Input: part model. Units: mm. Frame: model coordinates. Face numbers are marked on the shaded views. A direction names the side the tool comes from. Coordinates: 2 decimals unless noted, no trailing zeros. Order: outer loops, then holes, each group sorted by start corner. A loop starts at its lowest first (then second) coordinate and runs counter-clockwise, first axis right, second up. Notation, with made-up numbers: (47.25, -37.75) - (78.25, -37.75) arc R13 ccw to (78.25, -12.75) - close; hole circle Ø8 at (44, 9). An arc over 180 degrees is marked (long way). Use a Markdown table: item, result. Add a question column.
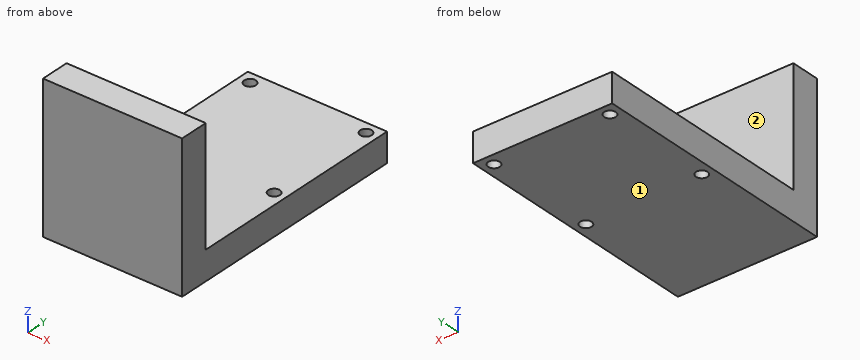
from build123d import *

# Parameters (mm, degrees)
SKETCH3_W           = 48
SKETCH3_H           = 30
SKETCH3_H_2         = 47
SKETCH3_R           = 2
SKETCH3_H_3         = 10
BOSS_EXTRUDE1_DEPTH = 10
SKETCH3_3_W         = 48
SKETCH3_3_H         = 10
BOSS_EXTRUDE2_DEPTH = 50


with BuildPart() as part:
    # Sketch3 → Boss-Extrude1 (new body)
    # profile 1 of 3: a face of its own
    with BuildSketch(Plane.XY):
        with Locations((0, -38.5)):
            Rectangle(SKETCH3_W, SKETCH3_H)
    # profile 2 of 3: a face of its own
    with BuildSketch(Plane.XY):
        Rectangle(SKETCH3_W, SKETCH3_H_2)
        with Locations((-20, 19.5)):
            Circle(SKETCH3_R, mode=Mode.SUBTRACT)
        with Locations((-20, -19.5)):
            Circle(SKETCH3_R, mode=Mode.SUBTRACT)
        with Locations((20, -19.5)):
            Circle(SKETCH3_R, mode=Mode.SUBTRACT)
        with Locations((20, 19.5)):
            Circle(SKETCH3_R, mode=Mode.SUBTRACT)
    # profile 3 of 3: a face of its own
    with BuildSketch(Plane.XY):
        with Locations((0, -58.5)):
            Rectangle(SKETCH3_W, SKETCH3_H_3)
    extrude(amount=BOSS_EXTRUDE1_DEPTH)

    # Sketch3_3 → Boss-Extrude2 (add)
    with BuildSketch(Plane.XY):
        with Locations((0, -58.5)):
            Rectangle(SKETCH3_3_W, SKETCH3_3_H)
    extrude(amount=BOSS_EXTRUDE2_DEPTH)


solid = part.part
1) Cut plane B-B (y = -19.5). Return the cut outline in (x, z).
2) Cut plane C-C (x = -7.5). Return the cut outline in (y, z), and give its area (3 significant figures).
3) Cut plane A-A (x = -20). Return the cut outline in (y, z), and give its area (3 significant figures).
4) Reachability of the marked faces 1 and 2 from +Z, -Z, +X, -X, +Y, -Y: full face, straight path, thin tool, end or side. Return the list, or none.
5) Material intervals for L1, parallel to Y at x = -20, z = 3.5; L2, parallel to X at y = 19, z = 4; L3, parallel to Z at x = -1.5, y = -50.5, sorted ascending.
6) Cut plane D-D (z = 38). Return the cut outline in (x, y), and give its area (3 significant figures).
7) Contact query for flat-ended pins moving along their axis: P1, Ø3, axis at x = 12.5, y = -54, coming from the -Z side; P2, Ø5, axis at x = 18, y = -13.5, coming from the +Z side; P3, Ø20, axis at x = 5.5, z = 37.5, coming from the +Y side; P4, Ø3.5, axis at x = -20, y = 19.5, coming from the -Z side. Output: stop coordinate, or through.
Computed:
| question | item | result |
|---|---|---|
| 1 | outline | (-24, 0) - (-22, 0) - (-22, 10) - (-24, 10) - close; (-18, 0) - (18, 0) - (18, 10) - (-18, 10) - close; (22, 0) - (24, 0) - (24, 10) - (22, 10) - close |
| 2 | outline | (-63.5, 0) - (23.5, 0) - (23.5, 10) - (-53.5, 10) - (-53.5, 50) - (-63.5, 50) - close |
| 2 | area | 1,270 mm2 |
| 3 | outline | (-63.5, 0) - (-21.5, 0) - (-21.5, 10) - (-53.5, 10) - (-53.5, 50) - (-63.5, 50) - close; (-17.5, 0) - (17.5, 0) - (17.5, 10) - (-17.5, 10) - close; (21.5, 0) - (23.5, 0) - (23.5, 10) - (21.5, 10) - close |
| 3 | area | 1,190 mm2 |
| 4 | face 1 | -Z, +X, -X, +Y, -Y |
| 4 | face 2 | +Z, +X, -X, +Y |
| 5 | L1 | y = -63.5 to -21.5, -17.5 to 17.5, 21.5 to 23.5 |
| 5 | L2 | x = -24 to -21.94, -18.06 to 18.06, 21.94 to 24 |
| 5 | L3 | z = 0 to 10 |
| 6 | outline | (-24, -63.5) - (24, -63.5) - (24, -53.5) - (-24, -53.5) - close |
| 6 | area | 480 mm2 |
| 7 | P1 | stops at z = 0 |
| 7 | P2 | stops at z = 10 |
| 7 | P3 | stops at y = -53.5 |
| 7 | P4 | passes through |
